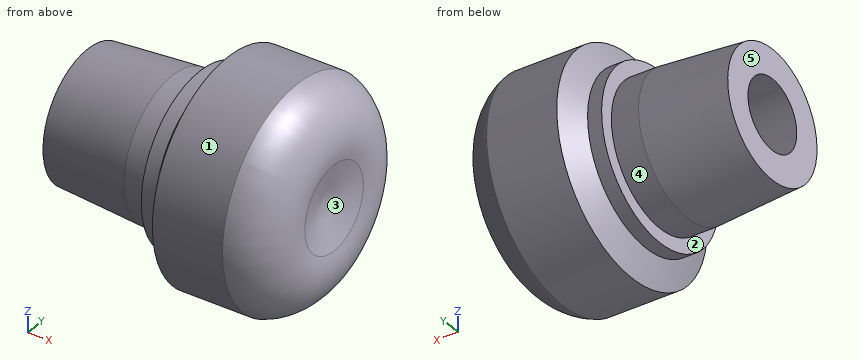
from build123d import *


with BuildPart() as f1:
    # F0 (on Front) → F1 (revolve)
    with BuildSketch(Plane.XZ):
        with BuildLine():
            Line((-114.3, 58.114587), (-114.3, 31.75))
            Line((-114.3, 31.75), (4.380015, 31.75))
            Line((4.380015, 31.75), (15.378538, 38.1))
            Line((15.378538, 38.1), (28.078538, 38.1))
            Line((28.078538, 38.1), (34.428538, 31.75))
            Line((34.428538, 31.75), (34.428538, 0))
            Line((34.428538, 0), (98.73198, 0))
            Line((98.73198, 0), (108.940844, 38.1))
            ThreePointArc((108.940844, 38.1), (104.562064, 74.670998), (76.148301, 98.1075))
            Line((76.148301, 98.1075), (12.648301, 98.1075))
            Line((12.648301, 98.1075), (0, 76.2))
            Line((0, 76.2), (-12.7, 76.2))
            Line((-12.7, 76.2), (-12.7, 63.5))
            Line((-12.7, 63.5), (-37.28501, 63.5))
            Line((-37.28501, 63.5), (-114.3, 58.114587))
        make_face()
    revolve(axis=Axis((50.931664, 0, 0), (1, 0, 0)))


solid = f1.part
Check sheet for the modelled part. Datum: model origin and axes. Units: mm. Face numbers are marked on the shaded views. A direction names the side the tool comes from. Coordinates: 2 decimals unless noted, no trailing zeros. Loops run counter-clockwise (first coordinate to the right, second up) from the corner with the lowest first, then second, coordinate; pieces in that order, holes last. Notation, with made-up numbers: (65, -3) -> (97, -3) arc R24 cw to (97, 35) -> close; hole circle Ø8 at (-18.75, 83). An arc over 180 degrees is marked (long way). Write item = value, one per line. Start each with the question number.
1. Material ranges on line 1 (Y direction, x = 19, z = 0); line 2 (Z direction, x = -35, y = 0), recorded low to high.
2. Depth check by flat-ended pin: P1, Ø1.5, axis at y = 74.5, z = -11, coming from the -X side; P2, Ø3, axis at x = -43.5, z = -52.5, coming from the +Y side; P3, Ø6, axis at x = 79.5, z = -10, coming from the +Y side. Enter the tip coordinate at first touch or a pass-through.
3. Tool access check on the marked faces 4 and 5. Record the directions out of +Z, -Z, +X, -X, +Y, -Y that give a thin tool (end or side, any length) a straight path to the whole face; none if there is none.
4. Draft check along Y on the marked faces 1, 2 and 3. Enter one of: released by +Y, released by -Y, zero draft, split by the parting line, or undercut.
5. Section check A-A on x = -86. Record the cut outline in (y, z).
Responses:
q1.line_1 = -98.11 to -38.1, 38.1 to 98.11
q1.line_2 = -63.5 to -31.75, 31.75 to 63.5
q2.P1 = -12.7
q2.P2 = 37.11
q2.P3 = 97.53
q3.face_4 = -X
q3.face_5 = +Z, -Z, -X, +Y, -Y
q4.face_1 = split by the parting line
q4.face_2 = zero draft
q4.face_3 = undercut
q5.outline = circle Ø120.19 at (0, 0); hole circle Ø63.5 at (0, 0)
